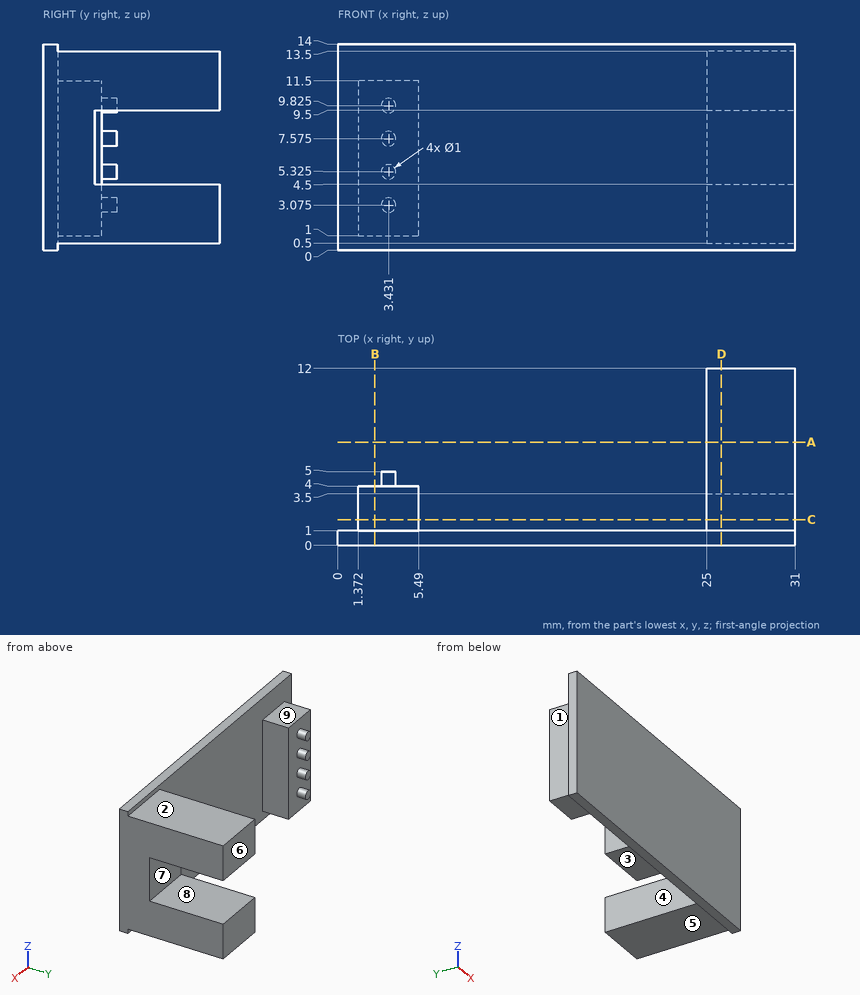
Could you check a few things on this drawing? It's one solid part, dimensions in mm from its lowest x, y, z. A direction names the side the tool comes from. Give positions to 0.01 mm unless a question says otherwise; leave off trailing zeros. Order: outer loops, then holes, each group sorted by start corner. A loop starts at its lowest first (then second) coordinate and runs counter-clockwise, first axis right, second up. Notation, with made-up numbers: (79.25, 75) - (136.25, 75) arc R24 ccw to (136.25, 91) - close; hole circle Ø3 at (47, 55.5). An arc over 180 degrees is marked (long way). Answer as a JSON object with one key per item and string values. Group by question number.
Item 1: Which directions (+Z, -Z, +X, -X, +Y, -Y) give clear straight access to the entire face, cutting with the end or side of a thin tool? Please do the marked faces 1, 2, 3, 4 and 5.
Item 2: If we section it at B-B on x = 2.5: Please give me the cut outline in (y, z).
Item 3: If we section it at A-A on y = 7: Please give me the cut outline in (x, z).
Item 4: If we mould it in two halves opening along Z, with no side actions, what happens to the marked faces 6, 7, 8 and 9? For each: pulls with the +Z half, pulls with the -Z half, needs draft (parallel to the pull), parting line crosses it, or undercut.
Item 5: For P1, Ø6, axis at x = 17, z = 5.5, coming from the +Y side; P2, Ø0.5, axis at x = 3.5, z = 10, coming from the +Y side; P3, Ø1.5, axis at x = 2.5, y = 2, coming from the -Z side, each with a flat end and sliding along its axis, tell me the tip position at first contact or that it passes through.
Item 6: Please list where these lines run through material, in increasing order: probe 1 along X at (y, z) = (1.5, 7.75); probe 2 along Z at (x, y) = (27, 9.75); probe 3 along Y at (x, z) = (10.5, 7).
Item 7: If we section it at C-C on y = 1.75: Please give me the cut outline in (x, z).
Item 8: If we section it at D-D on x = 26: Please give me the cut outline in (y, z).
Result set:
{
 "1": {"face 1": "+Z, -Z, -X, +Y", "face 2": "+Z, +X, -X, +Y", "face 3": "+X, +Y", "face 4": "+Z, -Z, +Y", "face 5": "-Z, +X, -X, +Y"},
 "2": {"outline": "(0, 0) - (1, 0) - (1, 1) - (4, 1) - (4, 11.5) - (1, 11.5) - (1, 14) - (0, 14) - close"},
 "3": {"outline": "(25, 0.5) - (31, 0.5) - (31, 4.5) - (25, 4.5) - close; (25, 9.5) - (31, 9.5) - (31, 13.5) - (25, 13.5) - close"},
 "4": {"face 6": "needs draft", "face 7": "undercut", "face 8": "undercut", "face 9": "pulls with the +Z half"},
 "5": {"P1": "y = 1", "P2": "y = 5", "P3": "z = 1"},
 "6": {"probe 1": "1.37 to 5.49, 25 to 31", "probe 2": "0.5 to 4.5, 9.5 to 13.5", "probe 3": "0 to 1"},
 "7": {"outline": "(1.37, 1) - (5.49, 1) - (5.49, 11.5) - (1.37, 11.5) - close; (25, 0.5) - (31, 0.5) - (31, 13.5) - (25, 13.5) - close"},
 "8": {"outline": "(0, 0) - (1, 0) - (1, 0.5) - (12, 0.5) - (12, 4.5) - (3.5, 4.5) - (3.5, 9.5) - (12, 9.5) - (12, 13.5) - (1, 13.5) - (1, 14) - (0, 14) - close"}
}
